Autodesk Inventor part; units mm, degrees
ref_plane "YZ Plane" through (0, 0, 0) normal (1, 0, 0) x (0, 1, 0)
ref_plane "XZ Plane" through (0, 0, 0) normal (0, 1, 0) x (-1, 0, 0)
ref_plane "XY Plane" through (0, 0, 0) normal (0, 0, 1) x (1, 0, 0)
sketch "Szkic1" plane through (0, 0, 0) normal (0, 0, 1) x (1, 0, 0)
  circle A0 centre (0, 0) radius 2.25
  circle A1 centre (0, 0) radius 3
  dimension "d0" = 4.5
  dimension "d1" = 6
extrude "Wyciągnięcie proste1" add sketch "Szkic1" against normal blind 1
sketch "Szkic4" plane through (0, 0, 0) normal (0, 0, 1) x (1, 0, 0)
  circle A0 centre (0, 0) radius 2.25
  circle A1 centre (0, 0) radius 3
  circle A2 centre (0, 0) radius 3
  circle A3 centre (0, 0) radius 2.25
  circle A4 centre (0, 0) radius 3.65
  line L0 (0, 0) -> (0, 8.5)
  circle A5 centre (0, 0) radius 2.4
  line L1 (0, 8.5) -> (0, 9.5)
  line L2 (0, 8.5) -> (5.1877, 8.5) construction
  line L3 (0, 9.5) -> (0, 10)
  line L4 (0, 10) -> (1.1899, 3.4506)
  line L5 (0, 10) -> (-1.1899, 3.4506)
  line L6 (-3.8268, 9.2388) -> (-0.2212, 3.6433)
  line L7 (-3.8268, 9.2388) -> (-2.4198, 2.7326)
  line L8 (-7.0711, 7.0711) -> (-1.5985, 3.2813)
  line L9 (-7.0711, 7.0711) -> (-3.2813, 1.5985)
  line L10 (-9.2388, 3.8268) -> (-2.7326, 2.4198)
  line L11 (-9.2388, 3.8268) -> (-3.6433, 0.2212)
  line L12 (-10, 0) -> (-3.4506, 1.1899)
  line L13 (-10, 0) -> (-3.4506, -1.1899)
  line L14 (-9.2388, -3.8268) -> (-3.6433, -0.2212)
  line L15 (-9.2388, -3.8268) -> (-2.7326, -2.4198)
  line L16 (-7.0711, -7.0711) -> (-3.2813, -1.5985)
  line L17 (-7.0711, -7.0711) -> (-1.5985, -3.2813)
  line L18 (-3.8268, -9.2388) -> (-2.4198, -2.7326)
  line L19 (-3.8268, -9.2388) -> (-0.2212, -3.6433)
  line L20 (0, -10) -> (-1.1899, -3.4506)
  line L21 (0, -10) -> (1.1899, -3.4506)
  line L22 (3.8268, -9.2388) -> (0.2212, -3.6433)
  line L23 (3.8268, -9.2388) -> (2.4198, -2.7326)
  line L24 (7.0711, -7.0711) -> (1.5985, -3.2813)
  line L25 (7.0711, -7.0711) -> (3.2813, -1.5985)
  line L26 (9.2388, -3.8268) -> (2.7326, -2.4198)
  line L27 (9.2388, -3.8268) -> (3.6433, -0.2212)
  line L28 (10, 0) -> (3.4506, -1.1899)
  line L29 (10, 0) -> (3.4506, 1.1899)
  line L30 (9.2388, 3.8268) -> (3.6433, 0.2212)
  line L31 (9.2388, 3.8268) -> (2.7326, 2.4198)
  line L32 (7.0711, 7.0711) -> (3.2813, 1.5985)
  line L33 (7.0711, 7.0711) -> (1.5985, 3.2813)
  line L34 (3.8268, 9.2388) -> (2.4198, 2.7326)
  line L35 (3.8268, 9.2388) -> (0.2212, 3.6433)
  point P0 (-0.9495, 4.7736)
  point P1 (-2.704, 4.0469)
  point P2 (-4.0469, 2.704)
  point P3 (-4.7736, 0.9495)
  point P4 (-4.7736, -0.9495)
  point P5 (-4.0469, -2.704)
  point P6 (-2.704, -4.0469)
  point P7 (-0.9495, -4.7736)
  point P8 (0.9495, -4.7736)
  point P9 (2.704, -4.0469)
  point P10 (4.0469, -2.704)
  point P11 (4.7736, -0.9495)
  point P12 (4.7736, 0.9495)
  point P13 (4.0469, 2.704)
  point P14 (2.704, 4.0469)
  point P15 (0.9495, 4.7736)
  dimension "d29" = 7.3
  dimension "d44" = 8.5
  dimension "d50" = 4.8
  dimension "d51" = 1
  dimension "d76" = 0.5
  dimension "d79" = 360
extrude "Wyciągnięcie proste4" add sketch "Szkic4" along normal blind 4 contours A5 | A1 | A4 | A4 L6 L5 L3 L1 L0 | L0 L1 L3 L4 L35 A4 | L35 L4 A4 | A4 L5 L6 | L4 L35 L34 L33 A4 | A4 L8 L7 L6 L5 | L33 L34 A4 | A4 L7 L8 | L34 L33 L32 L31 A4 | A4 L10 L9 L8 L7 | L31 L32 A4 | A4 L9 L10 | L32 L31 L30 L29 A4 | A4 L12 L11 L10 L9 | L29 L30 A4 | A4 L11 L12 | L30 L29 L28 L27 A4 | A4 L14 L13 L12 L11 | A4 L13 L14 | L27 L28 A4 | L27 L26 L25 A4 L28 | A4 L16 L15 L14 L13 | A4 L15 L16 | L25 L26 A4 | L25 L24 L23 A4 L26 | A4 L18 L17 L16 L15 | A4 L17 L18 | L23 L24 A4 | L23 L22 L21 A4 L24 | A4 L20 L19 L18 L17 | A4 L19 L20 | L21 L22 A4 | L21 L20 L19 A4 L22
sketch "Szkic5" plane through (0, 0, 4) normal (0, 0, 1) x (1, 0, 0)
  circle A0 centre (0, 0) radius 2.35
  dimension "d41" = 4.7
extrude "Wyciągnięcie proste5" cut sketch "Szkic5" against normal through all
sketch "Szkic6" plane through (0, 0, 4) normal (0, 0, 1) x (1, 0, 0)
  circle A0 centre (0, 0) radius 2.4
  dimension "d57" = 4.8
extrude "Wyciągnięcie proste6" cut sketch "Szkic6" against normal through all
ref_plane "Płaszczyzna konstrukcyjna1" through (0, 0, 0) normal (0, 0, -1) x (-1, 0, 0)
sketch "Szkic7" plane through (0, 0, 0) normal (0, 0, -1) x (-1, 0, 0)
  circle A0 centre (0, 0) radius 2.4
  circle A1 centre (0, 0) radius 1.5
  dimension "d61" = 3
extrude "Wyciągnięcie proste7" add sketch "Szkic7" against normal blind 1.2
properties part number "GEAR_SERV"
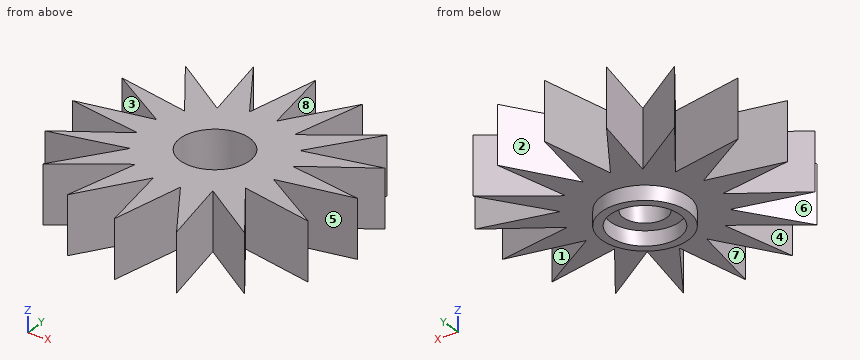
Geometry check sheet. Reference: the model listing, model coordinates, mm. Face numbers are marked on the shaded views. A direction names the side the tool comes from. Coordinates: 2 decimals unless noted, no trailing zeros. Loops run counter-clockwise (first coordinate to the right, second up) from the corner with the lowest first, then second, coordinate; pieces in that order, holes last. Notation, with made-up numbers: (-10.75, 78.25) - (42.25, 78.25) arc R7 cw to (42.25, 88.25) - close; hole circle Ø10 at (-9, 40.25). An arc over 180 degrees is marked (long way). Use one line per item in the form item = value. Start each with the question number.
Item 1: Mould release check, pull along X, two halves, no side actions. Record for the marked faces 1, 2, 3 and 4: +X half, -X half, draft (parallel to the pull), parting line (faces both ways), or undercut.
Item 2: Tool access check on the marked faces 5, 6, 7 and 8. Record the directions out of +Z, -Z, +X, -X, +Y, -Y that give a thin tool (end or side, any length) a straight path to the whole face; none if there is none.
Item 3: Section check D-D, the plane y = 8. Enter the section's corners in (x, z), and give its area (3 significant figures).
Item 4: Section check B-B, the plane y = 1.25. Enter the section's corners in (x, z), and give its area (3 significant figures).
Item 5: Gauge pin test, flat ends, axial feed: pin 1 (4 mm diameter, centred on x = 0, y = 0, fed in from -Z); pin 2 (3 mm diameter, centred on y = 7.5, z = -0.5, fed in from -X); pin 3 (2 mm diameter, centred on x = 7.5, z = 1, fed in from -Y). Record the tip position at first contact, or that the pin passes through.
Item 6: Section check C-C, the plane x = 6.25. Enter the section's corners in (y, z).
Item 7: Thickness scan on probe 1 along Y at (x, z) = (8.75, 2.8); probe 2 along Y at (x, z) = (0, -0.25); probe 3 along X at (y, z) = (6.5, 2.6). Record the ranges inside material, lowest first.
Computed:
q1.face_1 = +X half
q1.face_2 = undercut
q1.face_3 = -X half
q1.face_4 = undercut
q2.face_5 = +Z, -Z, +X
q2.face_6 = +Z, -Z
q2.face_7 = +Z, -Z, -Y
q2.face_8 = +Z, -Z, +Y
q3.outline = (-3.56, 0) - (-3.03, 0) - (-3.03, 4) - (-3.56, 4) - close; (-0.36, 0) - (0.36, 0) - (0.36, 4) - (-0.36, 4) - close; (3.03, 0) - (3.56, 0) - (3.56, 4) - (3.03, 4) - close
q3.area = 7.15 mm2
q4.outline = (-5.24, 0) - (-2.73, 0) - (-2.73, -1) - (-2.05, -1) - (-2.05, 0) - (-0.83, 0) - (-0.83, 1.2) - (-2.05, 1.2) - (-2.05, 4) - (-5.24, 4) - close; (0.83, 0) - (2.05, 0) - (2.05, -1) - (2.73, -1) - (2.73, 0) - (5.24, 0) - (5.24, 4) - (2.05, 4) - (2.05, 1.2) - (0.83, 1.2) - close
q4.area = 29.8 mm2
q5.pin_1 = 0
q5.pin_2 = -7.07
q5.pin_3 = -7.07
q6.outline = (-6.5, 0) - (-5.89, 0) - (-5.89, 4) - (-6.5, 4) - close; (-3.18, 0) - (-1.9, 0) - (-1.9, 4) - (-3.18, 4) - close; (-0.68, 0) - (0.68, 0) - (0.68, 4) - (-0.68, 4) - close; (1.9, 0) - (3.18, 0) - (3.18, 4) - (1.9, 4) - close; (5.89, 0) - (6.5, 0) - (6.5, 4) - (5.89, 4) - close
q7.probe_1 = -3.72 to -3.51, -0.23 to 0.23, 3.51 to 3.72
q7.probe_2 = -3 to -2.4, 2.4 to 3
q7.probe_3 = -6.68 to -6.25, -3.23 to -2.06, -0.64 to 0.64, 2.06 to 3.23, 6.25 to 6.68
